Autodesk Inventor part; units mm, degrees
ref_plane "YZ Plane" through (0, 0, 0) normal (1, 0, 0) x (0, 1, 0)
ref_plane "XZ Plane" through (0, 0, 0) normal (0, 1, 0) x (-1, 0, 0)
ref_plane "XY Plane" through (0, 0, 0) normal (0, 0, 1) x (1, 0, 0)
sketch "Sketch1" plane through (0, 0, 0) normal (0, 1, 0) x (-1, 0, 0)
  line L0 (0, 0) -> (600, 0)
  line L1 (600, 0) -> (600, -830)
  line L2 (600, -830) -> (0, -830)
  line L3 (0, -830) -> (0, 0)
  dimension "d0" = 600
  dimension "d1" = 830
extrude "Extrusion1" add sketch "Sketch1" along normal blind 500
shell "Shell1" thickness 10 removed faces 1 at (-200, 500, -276.6667)
equation "\"BendRadius\" = Thickness"
equation "\"BendReliefWidth\" = Thickness"
equation "\"BendReliefDepth\" = 0.5 * Thickness"
equation "\"CornerReliefSize\" = 4 * Thickness"
equation "\"MinimumRemnant\" = 2 * Thickness"
equation "\"TransitionRadius\" = BendRadius"
equation "\"JacobiRadiusSize\" = BendRadius"
equation "\"GapSize\" = Thickness"
properties part number "Paste Container"
Verification items for the finished model (mm, model axes). A direction names the side the tool comes from. Round coordinates to 2 decimals unless told otherwise and drop trailing zeros. Write each loop counter-clockwise with the first axis right and the second up, starting at its lowest first coordinate (ties: lowest second). Pieces come first, ordered by that corner, then holes.
1. Access from +Z, -Z, +X, -X, +Y, -Y to the whole of each face (thin tool, end or side, straight path). Record for faces 1 (the flat face through (-296, 246, 0)), 2 (the flat face through (-296, 10, -409)).
2. Section check C-C on x = -226. Enter the section's corners in (y, z).
3. Section check A-A on y = 272.5. Enter the section's corners in (x, z).
4. Scan lines: L1, parallel to Z at x = -334, y = 253; L2, parallel to X at y = 212, z = -187; L3, parallel to Y at x = -351.5, z = -101.5. Record each from-to range of solid material in increasing order.
5. Section check B-B on z = -471. Enter the section's corners in (x, y).
6. Gauge pin test, flat end, axial feed: P1, Ø6, axis at x = -438, z = -679.5, coming from the +Y side. Record the tip position at first contact, or that the pin passes through.
Answer:
1. face 1: +Z, +X, -X, +Y, -Y
1. face 2: +Y
2. outline: (0, -830) - (500, -830) - (500, -820) - (10, -820) - (10, -10) - (500, -10) - (500, 0) - (0, 0) - close
3. outline: (-600, -830) - (0, -830) - (0, 0) - (-600, 0) - close; hole (-590, -820) - (-10, -820) - (-10, -10) - (-590, -10) - close
4. L1: z = -830 to -820, -10 to 0
4. L2: x = -600 to -590, -10 to 0
4. L3: y = 0 to 10
5. outline: (-600, 0) - (0, 0) - (0, 500) - (-10, 500) - (-10, 10) - (-590, 10) - (-590, 500) - (-600, 500) - close
6. P1: stops at y = 10
